```python
from build123d import *

# Parameters (mm, degrees)
F1_DEPTH = 20
F2_R     = 10
F3_T     = -1
F4_W     = 28.581038
F4_H     = 2.5
F5_DEPTH = 1


with BuildPart() as f1:
    # F0 (on Top) → F1 (new body)
    with BuildSketch(Plane.XY):
        Polygon((-15, 50), (-50, -50), (50, -50), (15, 50), align=None)
    extrude(amount=F1_DEPTH)

    # F2
    f2_edges = [f1.edges().sort_by_distance(p)[0] for p in [
        (-50, -50, 10),
        (50, -50, 10),
    ]]
    fillet(f2_edges, radius=F2_R)

    # F3
    f3_openings = [f1.faces().sort_by_distance(p)[0] for p in [
        (0, -8.435574, 20),
    ]]
    offset(amount=F3_T, openings=f3_openings)

    # F4 (on face) → F5 (cut, through all)
    with BuildSketch(Plane.XZ.offset(-49)):
        with Locations((0, 2.25)):
            Rectangle(F4_W, F4_H)
    extrude(amount=-F5_DEPTH, mode=Mode.SUBTRACT)


solid = f1.part
```
Build history of the part. All positions in model axes, mm. A direction names the side the tool comes from. Round coordinates to 2 decimals unless told otherwise and drop trailing zeros. Write each loop counter-clockwise with the first axis right and the second up, starting at its lowest first coordinate (ties: lowest second). Pieces come first, ordered by that corner, then holes. Notation, with made-up numbers: (15.25, -28.75) - (67.25, -28.75) arc R14 ccw to (67.25, -20.75) - close; hole circle Ø10 at (-30.75, 79.25). An arc over 180 degrees is marked (long way). Write each question's results on one line, items separated by ' | '. Start each with the question number.
Item 1: Mould opens along Y. For faces 1 (the face through (0, 49, 12)), 2 (the face through (-1, -49, 10)), 3 (the face through (30.4, 6, 9.9)), 4 (the face through (-44.138, -45.677, 10.14)) say: pulls with the +Y half, pulls with the -Y half, needs draft (parallel to the pull), parting line crosses it, or undercut.
Item 2: Which spindle directions (+Z, -Z, +X, -X, +Y, -Y) get a long thin tool onto all of the face, cutting with end or side? Do faces 5 (the face through (29.556, 5.384, 10.367)), 6 (the face through (30.4, 3.9, 20)). Say none if no direction does.
Item 3: Saw through at D-D (x = 30.5). Write the cut outline in (y, z).
Item 4: Saw through at B-B (x = 0.5). Write the cut outline in (y, z).
Item 5: Saw through at C-C (y = 7). Write the cut outline in (x, z).
Item 6: Saw through at A-A (z = 13). Write the cut outline in (x, y), and give its area (3 significant figures).
Item 7: Drop flat-ended pins along their axis: P1, Ø0.5, axis at y = 49.5, z = 2, coming from the -X side; P2, Ø1, axis at y = 13.5, z = 17.5, coming from the -X side; P3, Ø0.8, axis at y = 49.5, z = 2, coming from the +X side (3 decimals). Give the stop position or say it passes through.
Item 8: Wall check: L1, parallel to Y at x = 6, z = 7.5; L2, parallel to Z at x = -6, y = -13; L3, parallel to X at y = -39, z = 4.5. Give the ranges that are in metal, low to high. Write a range as [from, to].
Results are:
1) face 1: undercut | face 2: undercut | face 3: pulls with the +Y half | face 4: parting line crosses it
2) face 5: +Z | face 6: +Z, +X, -X, +Y, -Y
3) outline: (-50, 0) - (5.71, 0) - (5.71, 20) - (2.69, 20) - (2.69, 1) - (-49, 1) - (-49, 20) - (-50, 20) - close
4) outline: (-50, 0) - (50, 0) - (50, 1) - (-49, 1) - (-49, 20) - (-50, 20) - close; (49, 3.5) - (50, 3.5) - (50, 20) - (49, 20) - close
5) outline: (-30.05, 0) - (30.05, 0) - (30.05, 20) - (28.99, 20) - (28.99, 1) - (-28.99, 1) - (-28.99, 20) - (-30.05, 20) - close
6) outline: (-45.34, -36.7) arc R10 ccw to (-35.91, -50) - (35.91, -50) arc R10 ccw to (45.34, -36.7) - (15, 50) - (-15, 50) - close; hole (-44.4, -37.03) arc R9 ccw to (-35.91, -49) - (35.91, -49) arc R9 ccw to (44.4, -37.03) - (14.29, 49) - (-14.29, 49) - close | area: 320 mm²
7) P1: stops at x = -15.26 | P2: stops at x = -27.95 | P3: stops at x = 15.315
8) L1: y = [-50, -49], [49, 50] | L2: z = [0, 1] | L3: x = [-45.86, -44.85], [44.85, 45.86]
